Source: three-view drawing plus pictorial views. Frame: mm from the lowest corner of the part. Coordinates: 2 decimals unless noted, no trailing zeros. Write each loop counter-clockwise with the first axis right and the second up, starting at its lowest first coordinate (ties: lowest second). Pieces come first, ordered by that corner, then holes. Notation, with made-up numbers: (-28.75, 86) - (30.25, 86) arc R16 cw to (30.25, 115) - close; hole circle Ø8 at (18.25, 47.5). An arc over 180 degrees is marked (long way). Put each result on its own line as item: value. Start each with the question number.
1. Line query: line 1 (Y direction, x = 139.5, z = 2.25); line 2 (Z direction, x = 86, y = 7.25); line 3 (Y direction, x = 23, z = 6.5). Output: solid intervals per line, ascending.
2. Cut plane C-C, the plane y = 9. Return loops of the section in (x, z).
3. Pin query (flat end, axial travel): pin 1 (1 mm diameter, centred on x = 186, z = 5.5, fed in from -Y); pin 2 (0.8 mm diameter, centred on x = 118, y = 5.5, fed in from +Z). Return the tip coordinate at first contact, or that it passes through.
4. Cut plane B-B, the plane x = 50. Return loops of the section in (y, z).
5. Cut plane A-A, the plane z = 5.5. Return loops of the section in (x, y), and give its area (3 significant figures).
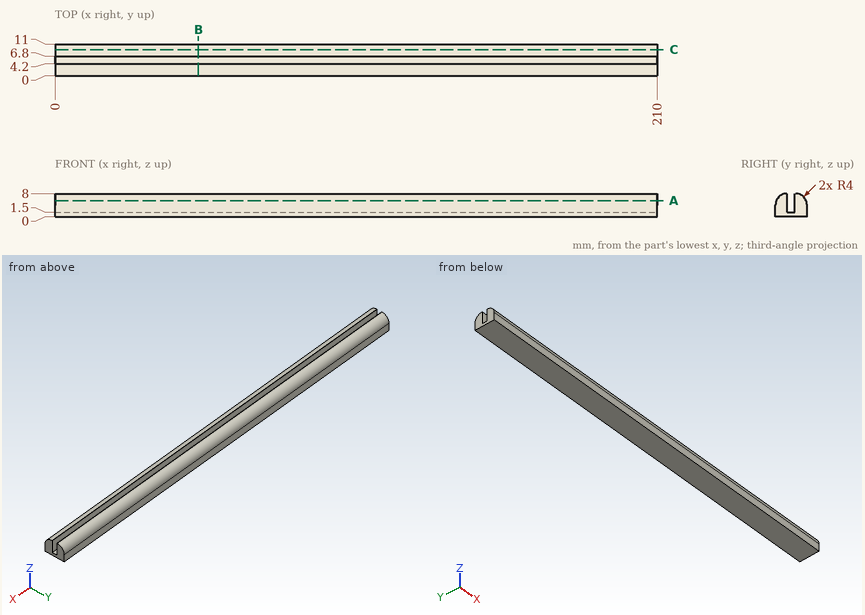
Report:
1. line 1: y = 0 to 4.2, 6.8 to 11
1. line 2: z = 0 to 7.99
1. line 3: y = 0.88 to 4.2, 6.8 to 10.12
2. outline: (0, 0) - (210, 0) - (210, 7.46) - (0, 7.46) - close
3. pin 1: stops at y = 0.13
3. pin 2: stops at z = 1.5
4. outline: (0, 0) - (11, 0) - (11, 4) arc R4 ccw to (7, 8) - (6.8, 8) - (6.8, 1.5) - (4.2, 1.5) - (4.2, 8) - (4, 8) arc R4 ccw to (0, 4) - close
5. outline: (0, 0.29) - (210, 0.29) - (210, 4.2) - (0, 4.2) - close; (0, 6.8) - (210, 6.8) - (210, 10.71) - (0, 10.71) - close
5. area: 1,640 mm^2
